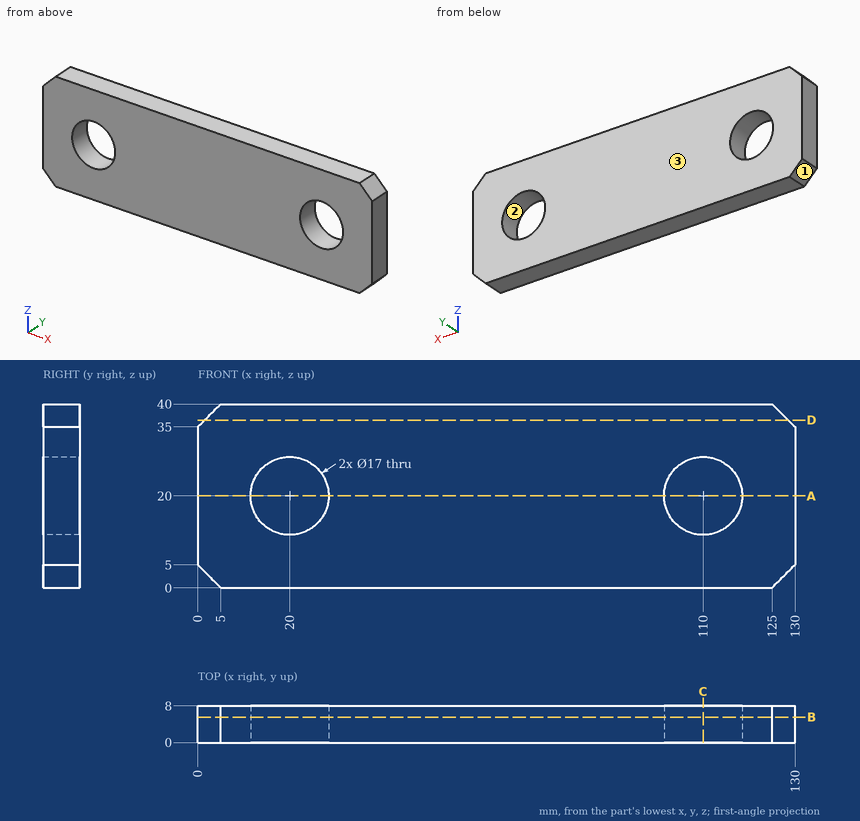
Answer from the drawing. Dimensions are ordinates in mm from the lowest x, y and z of the part. Coordinates: 2 decimals unless noted, no trailing zeros. Write each loop counter-clockwise with the first axis right and the second up, starting at its lowest first coordinate (ties: lowest second). Pieces come first, ordered by that corner, then holes. Notation, with made-up numbers: M 26.25,7 L 46.25,7 A25 cw 46.25,35 Z; hole C -4,86 d2. An arc over 180 degrees is marked long. Write item = value, one per line.
1. Determine the mould class of the marked faces 1, 2 and 3 for opening direction X: released by +X, released by -X, zero draft, split by the parting line, or undercut.
Solution:
face_1 = released by -X
face_2 = undercut
face_3 = zero draft
2. The part is cut by section D-D (z = 36.5). Determine the outline of the cut face in (x, y), then the cut area to 3 significant figures.
Solution:
outline = M 1.5,0 L 128.5,0 L 128.5,8 L 1.5,8 Z
area = 1,020 mm2
3. The part is cut by section C-C (x = 110). Determine the outline of the cut face in (y, z), then the cut area to 3 significant figures.
Solution:
outline = M 0,0 L 8,0 L 8,11.5 L 0,11.5 Z; M 0,28.5 L 8,28.5 L 8,40 L 0,40 Z
area = 184 mm2
4. The part is cut by section A-A (z = 20). Determine the outline of the cut face in (x, y), then the cut area to 3 significant figures.
Solution:
outline = M 0,0 L 11.5,0 L 11.5,8 L 0,8 Z; M 28.5,0 L 101.5,0 L 101.5,8 L 28.5,8 Z; M 118.5,0 L 130,0 L 130,8 L 118.5,8 Z
area = 768 mm2
5. The part is cut by section B-B (y = 5.5). Determine the outline of the cut face in (x, z).
Solution:
outline = M 0,5 L 5,0 L 125,0 L 130,5 L 130,35 L 125,40 L 5,40 L 0,35 Z; hole C 20,20 d17; hole C 110,20 d17
6. Straight lines are drawn through the part: line 1 (X direction, y = 5.5, z = 20); line 2 (X direction, y = 6.75, z = 12.5); line 3 (Z direction, x = 24.5, y = 2.5). For each, find the intervals that lie inside material, in ascending order. Write a range as from..to.
Solution:
line_1 = 0..11.5, 28.5..101.5, 118.5..130
line_2 = 0..16, 24..106, 114..130
line_3 = 0..12.79, 27.21..40
7. Flat-ended cylindrical pins translate along their axes: pin 1 (2 mm diameter, centred on x = 63, z = 19, fed in from -Y); pin 2 (10 mm diameter, centred on x = 20, z = 20, fed in from -Y). Find the tip coordinate at first contact, or state that the pin passes through.
Solution:
pin_1 = 0
pin_2 = through
